Build history of the part. All positions in model axes, mm. A direction names the side the tool comes from. Give positions to 0.01 mm unless a question says otherwise; leave off trailing zeros. Loops run counter-clockwise (first coordinate to the right, second up) from the corner with the lowest first, then second, coordinate; pieces in that order, holes last. Notation, with made-up numbers: M 5,48 L 19,48 A19 ccw 19,85 Z; hole C 58.25,49.25 d4. An arc over 180 degrees is marked long. Answer as a JSON object with one key per item and string values. Group by question number.
1. Slice it at A-A (y = -23). List the corners of the cut face in (x, z), then the cut area to 3 significant figures.
2. Slice it at B-B (x = 27). List the corners of the cut face in (y, z), then the cut area to 3 significant figures.
3. Mould opens along Z. For faces 1 (the face through (15.567, -19.759, -0.13)), 2 (the face through (67.856, -19, 0)), 3 (the face through (37.414, -6.872, -0.912)) say: released by +Z, released by -Z, zero draft, split by the parting line, or undercut.
4. Slice it at C-C (z = 5.5). List the corners of the cut face in (x, y).
5. Drill centre lines: line 1 along Y through (x, z) = (20, 9.25); line 2 along Z through (x, y) = (14.5, -24); line 3 along Z through (x, y) = (59.5, -1.5). Where is each one in solid material? Low to high. Write a range as [from, to].
6. Drop flat-ended pins along their axis: pin 1 Ø8 at (x, z) = (57.98, 0) entering from +Y; pin 2 Ø4 at (x, z) = (40.5, -0.5) entering from +Y; pin 3 Ø8 at (x, z) = (32, 2.5) entering from +Y; pin 4 Ø11.5 at (x, z) = (50.5, 9.5) entering from +Y. Give the stop position or say it passes through.
7. 3-axis set-ups, long thin cutter, end or side, ignore diameter. For faces 4 (the face through (37, -8, 7)), 5 (the face through (18.29, -29.38, 0.96)), 6 (the face through (37, -19, -12.5)): which of +Z, -Z, +X, -X, +Y, -Y reach the whole face in a straight line?
from build123d import *

# Parameters (mm, degrees)
SKETCH1_W             = 61.75
SKETCH1_H             = 38
BOSS_EXTRUDE1_DEPTH   = 12.5
CUT_EXTRUDE1_REACH    = 75.575
FILLET1_R             = 1
M6_TAPPED_HOLE1_D     = 5
M6_TAPPED_HOLE1_DEPTH = 17
M6_TAPPED_HOLE1_TIP   = 1.502151548


with BuildPart() as part:
    # Sketch1 → Boss-Extrude1 (new, symmetric)
    with BuildSketch(Plane.XY):
        with Locations((36.981465557, -19)):
            Rectangle(SKETCH1_W, SKETCH1_H)
    extrude(amount=BOSS_EXTRUDE1_DEPTH, both=True)

    # Sketch2 → Cut-Extrude1 (cut, up to next)
    with BuildSketch(Plane(origin=(67.856465557, 0, 0), x_dir=(0, 0, -1), z_dir=(1, 0, 0)), mode=Mode.PRIVATE) as cut_extrude1_sk1:
        with BuildLine():
            Line((2.342754418, 0), (2.122152056, -4.209343825))
            ThreePointArc((2.122152056, -4.209343825), (0.88105222, -6.901497484), (-1.872366083, -8))
            Line((-1.872366083, -8), (-12.5, -8))
            Line((-12.5, -8), (-12.5, 0))
            Line((-12.5, 0), (2.342754418, 0))
        make_face()
    cut_extrude1_tool1 = extrude(cut_extrude1_sk1.sketch, amount=-CUT_EXTRUDE1_REACH, mode=Mode.PRIVATE) & part.part
    add(cut_extrude1_tool1.solids().sort_by_distance((67.856466, -3.896267, 5.35091))[0], mode=Mode.SUBTRACT)

    # Fillet1
    fillet1_edges = [part.edges().sort_by_distance(p)[0] for p in [
        (36.981465557, 0, -2.342754418),
    ]]
    fillet(fillet1_edges, radius=FILLET1_R)

    # M6 Tapped Hole1
    with Locations(Plane(origin=(0, -38, 0), x_dir=(-1, 0, 0), z_dir=(0, -1, 0))):
        with Locations((-57.981465557, 0), (-15.981465557, 0)):
            Hole(M6_TAPPED_HOLE1_D / 2, depth=M6_TAPPED_HOLE1_DEPTH)
            with Locations((0, 0, -(M6_TAPPED_HOLE1_DEPTH + M6_TAPPED_HOLE1_TIP / 2))):  # 118° drill point
                Cone(0, M6_TAPPED_HOLE1_D / 2, M6_TAPPED_HOLE1_TIP, mode=Mode.SUBTRACT)


solid = part.part
Established:
{
 "1": {"outline": "M 6.11,-12.5 L 67.86,-12.5 L 67.86,12.5 L 6.11,12.5 Z; hole C 15.98,0 d5; hole C 57.98,0 d5", "area": "1,500 mm^2"},
 "2": {"outline": "M -38,-12.5 L 0,-12.5 L 0,-3.29 A1 ccw -0.95,-2.29 L -4.21,-2.12 A4 cw -8,1.87 L -8,12.5 L -38,12.5 Z", "area": "836 mm^2"},
 "3": {"face 1": "undercut", "face 2": "zero draft", "face 3": "released by +Z"},
 "4": {"outline": "M 6.11,-38 L 67.86,-38 L 67.86,-8 L 6.11,-8 Z"},
 "5": {"line 1": "y = [-38, -8]", "line 2": "z = [-12.5, -2.01], [2.01, 12.5]", "line 3": "z = [-12.5, -2.26]"},
 "6": {"pin 1": "stops at y = 0", "pin 2": "stops at y = -0.39", "pin 3": "stops at y = -6.15", "pin 4": "stops at y = -8"},
 "7": {"face 4": "+Z, +X, -X, +Y", "face 5": "-Y", "face 6": "-Z, +X, -X, +Y, -Y"}
}
